CAD build for the part. Positions are in the model's coordinates, mm. Face numbers are marked on the shaded views. A direction names the side the tool comes from. Coordinates: 2 decimals unless noted, no trailing zeros. Write item = value, one per line. Start each with the question number.
(1) Pull direction Z, two halves, no side cores. Call the marked faces 1, 2, 3 and 4: +Z half, -Z half, draft (parallel to the pull), parting line (faces both ways), or undercut.
(2) Band-saw the part on A-A (x = 0). Count the separate pieces of the cut face and the enclosed holes in it, and give its area (3 significant figures).
(3) Drill centre lines: line 1 (X direction, y = 2, z = 5.3); line 2 (X direction, y = 1, z = -5.5); line 3 (X direction, y = 2.9, z = 3.5). Where is each one in solid material? Low to high. Write a range as from..to.
(4) Flat gauge pins, fed straight in: P1, Ø0.8, axis at x = -2.5, z = 5, coming from the +Y side; P2, Ø2.5, axis at x = -1.5, y = 2.5, coming from the -Z side; P3, Ø1, axis at y = 2, z = 2.5, coming from the -X side. Where does each tip first touch, or does it go through?
(5) Tool access for the marked faces 5, 6, 7, 8 and 9: list every direction of +Z, -Z, +X, -X, +Y, -Y with a clear straight run to the whole face (end or side of a thin tool).
```python
from build123d import *

# Parameters (mm, degrees)
FILLET1_R               = 1.5
SKETCH4_W               = 2.4
SKETCH4_H               = 4.5
SKETCH4_W_2             = 2.5
SKETCH4_W_3             = 8
SKETCH4_H_2             = 3.5
CUT_EXTRUDE1_DEPTH      = 3.5
SKETCH3_W               = 7.5
SKETCH3_H               = 6
CUT_EXTRUDE2_DEPTH      = 12.470832747
CUT_EXTRUDE5_DEPTH      = 11.900917559
CUT_EXTRUDE5_DEPTH_BACK = 1
SKETCH5_R               = 2
CUT_EXTRUDE6_START      = -0.5
CUT_EXTRUDE6_DEPTH      = 1.5
SKETCH9_W               = 1
SKETCH9_H               = 3
CUT_EXTRUDE9_DEPTH      = 12.470832747


with BuildPart() as part:
    # Sketch1 → Loft1 section 0
    with BuildSketch(Plane(origin=(0, 0, 0), x_dir=(1, 0, 0), z_dir=(0, 1, 0))):
        with BuildLine():
            Line((-7.3, 7.3), (7.3, 7.3))
            Line((7.3, 7.3), (7.3, -7.3))
            Line((7.3, -7.3), (-7.3, -7.3))
            Line((-7.3, -7.3), (-7.3, 7.3))
        make_face()
    # Sketch2 → Loft1 section 1
    with BuildSketch(Plane(origin=(0, 5, 0), x_dir=(1, 0, 0), z_dir=(0, 1, 0))):
        with BuildLine():
            Line((-5.5, 6.5), (5.5, 6.5))
            Line((5.5, 6.5), (5.5, -4.5))
            Line((5.5, -4.5), (-5.5, -4.5))
            Line((-5.5, -4.5), (-5.5, 6.5))
        make_face()
    loft()

    # Fillet1
    fillet1_edges = [part.edges().sort_by_distance(p)[0] for p in [
        (0, 5, -6.5),
    ]]
    fillet(fillet1_edges, radius=FILLET1_R)

    # Sketch4 → Cut-Extrude1 (cut)
    with BuildSketch(Plane(origin=(0, 5, 0), x_dir=(1, 0, 0), z_dir=(0, 1, 0))):
        with Locations((-6.1, -5.05)):
            Rectangle(SKETCH4_W, SKETCH4_H)
        with Locations((6.05, 5.05)):
            Rectangle(SKETCH4_W_2, SKETCH4_H)
        with Locations((-6.1, 5.05)):
            Rectangle(SKETCH4_W, SKETCH4_H)
        with Locations((6.05, -5.05)):
            Rectangle(SKETCH4_W_2, SKETCH4_H)
        with Locations((0, -5.55)):
            Rectangle(SKETCH4_W_3, SKETCH4_H_2)
    extrude(amount=-CUT_EXTRUDE1_DEPTH, mode=Mode.SUBTRACT)

    # Shell2: read off the stored shape, not the designer's step
    # Shell2: loft between two sections, ruled curve by curve
    shell2_from = [
        Edge.make_line((5.705760369, 0, 1.3), (5.705760369, 0, -1.3)),
        Edge.make_line((-3.4, 0, -5.780921332), (3.3, 0, -5.780921332)),
        Edge.make_line((-5.705760369, 0, 1.3), (-5.705760369, 0, -1.3)),
        Edge.make_line((5.705760369, 0, -1.3), (3.3, 0, -1.3)),
        Edge.make_line((-5.705760369, 0, -1.3), (-3.4, 0, -1.3)),
        Edge.make_line((3.3, 0, -5.780921332), (3.3, 0, -1.3)),
        Edge.make_line((3.3, 0, 1.3), (3.3, 0, 2.3)),
        Edge.make_line((-3.4, 0, -5.780921332), (-3.4, 0, -1.3)),
        Edge.make_line((-3.4, 0, 2.3), (-3.4, 0, 1.3)),
        Edge.make_line((-3.4, 0, 1.3), (-5.705760369, 0, 1.3)),
        Edge.make_line((5.705760369, 0, 1.3), (3.3, 0, 1.3)),
        Edge.make_line((3.3, 0, 2.3), (-3.4, 0, 2.3)),
    ]
    shell2_to = [
        Edge.make_line((4.445760369, 3.5, 1.3), (4.445760369, 3.5, -1.3)),
        Edge.make_line((-3.4, 3.5, -5.220921332), (3.3, 3.5, -5.220921332)),
        Edge.make_line((-4.445760369, 3.5, 1.3), (-4.445760369, 3.5, -1.3)),
        Edge.make_line((4.445760369, 3.5, -1.3), (3.3, 3.5, -1.3)),
        Edge.make_line((-4.445760369, 3.5, -1.3), (-3.4, 3.5, -1.3)),
        Edge.make_line((3.3, 3.5, -5.220921332), (3.3, 3.5, -1.3)),
        Edge.make_line((3.3, 3.5, 1.3), (3.3, 3.5, 2.3)),
        Edge.make_line((-3.4, 3.5, -5.220921332), (-3.4, 3.5, -1.3)),
        Edge.make_line((-3.4, 3.5, 2.3), (-3.4, 3.5, 1.3)),
        Edge.make_line((-3.4, 3.5, 1.3), (-4.445760369, 3.5, 1.3)),
        Edge.make_line((4.445760369, 3.5, 1.3), (3.3, 3.5, 1.3)),
        Edge.make_line((3.3, 3.5, 2.3), (-3.4, 3.5, 2.3)),
    ]
    shell2 = Solid(Shell([*[Face.make_surface_from_curves(shell2_from[k], shell2_to[k]) for k in range(12)], Face(Wire(shell2_from)), Face(Wire(shell2_to))]))
    add(shell2, mode=Mode.SUBTRACT)

    # Sketch3 → Cut-Extrude2 (cut, through all)
    with BuildSketch(Plane.XZ):
        Rectangle(SKETCH3_W, SKETCH3_H)
    extrude(amount=-CUT_EXTRUDE2_DEPTH, mode=Mode.SUBTRACT)

    # Sketch5 → Cut-Extrude5 (cut, two sides: drawn at the far end of the back side and taken through both)
    with BuildSketch(Plane(origin=(0, 1.5, 0), x_dir=(1, 0, 0), z_dir=(0, 1, 0)).offset(-CUT_EXTRUDE5_DEPTH_BACK)):
        with Locations((0, -5.3)):
            Circle(SKETCH5_R)
    extrude(amount=CUT_EXTRUDE5_DEPTH + CUT_EXTRUDE5_DEPTH_BACK, mode=Mode.SUBTRACT)

    # Cut-Extrude6: read off the stored shape, not the designer's step
    # Cut-Extrude6 outline → Cut-Extrude6 (cut)
    with BuildSketch(Plane.XZ.offset(CUT_EXTRUDE6_START)):
        with BuildLine():
            Line((1.936491673, 5.8), (-1.936491673, 5.8))
            ThreePointArc((-1.936491673, 5.8), (-2, 5.3), (-1.936491673, 4.8))
            Line((-1.936491673, 4.8), (1.936491673, 4.8))
            ThreePointArc((1.936491673, 4.8), (2, 5.3), (1.936491673, 5.8))
        make_face()
    extrude(amount=CUT_EXTRUDE6_DEPTH, mode=Mode.SUBTRACT)

    # Sketch9 → Cut-Extrude9 (cut, through all)
    with BuildSketch(Plane(origin=(0, 0, 0), x_dir=(1, 0, 0), z_dir=(0, 1, 0))):
        with Locations((-5.4, 4.3)):
            Rectangle(SKETCH9_W, SKETCH9_H)
        with Locations((5.3, 4.3)):
            Rectangle(SKETCH9_W, SKETCH9_H)
        with Locations((-5.4, -4.3)):
            Rectangle(SKETCH9_W, SKETCH9_H)
        with Locations((5.3, -4.3)):
            Rectangle(SKETCH9_W, SKETCH9_H)
    extrude(amount=CUT_EXTRUDE9_DEPTH, mode=Mode.SUBTRACT)


solid = part.part
```
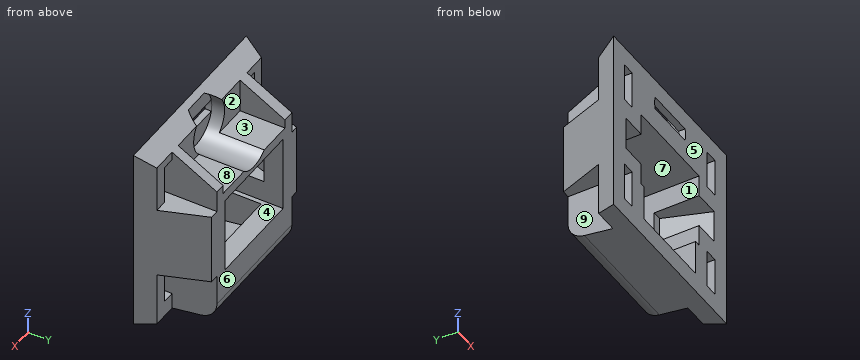
Findings below:
q1.face_1 = undercut
q1.face_2 = draft
q1.face_3 = +Z half
q1.face_4 = undercut
q2.separate_pieces = 3
q2.enclosed_holes = 0
q2.area = 13.3 mm²
q3.line_1 = -4.9..-4, 4..4.8
q3.line_2 = -6.94..-5.9, -4.9..-3.4, 3.3..4.8, 5.8..6.94
q3.line_3 = -4.9..-0.87, 0.87..4.8
q4.P1 = 1.5
q4.P2 = -7.1
q4.P3 = -6.76
q5.face_5 = +Z, -Z, +X, -X, -Y
q5.face_6 = +Z, -Z, +X, -X, +Y
q5.face_7 = +Y, -Y
q5.face_8 = +Z, +Y
q5.face_9 = +Y
